from build123d import *

# Parameters (mm, degrees)
SCHIZZO1_W                   = 170
SCHIZZO1_H                   = 55
ESTRUSIONE_ESTRUSIONE2_DEPTH = 5
SCHIZZO2_W                   = 15
SCHIZZO2_H                   = 5
TAGLIO_ESTRUSIONE1_DEPTH     = 6
TAGLIO_ESTRUSIONE3_DEPTH     = 6


with BuildPart() as part:
    # Schizzo1 → Estrusione-Estrusione2 (new body)
    with BuildSketch(Plane(origin=(0, 0, 0), x_dir=(1, 0, 0), z_dir=(0, 1, 0))):
        with Locations((30.43505086, -0.781075862)):
            Rectangle(SCHIZZO1_W, SCHIZZO1_H)
    extrude(amount=-ESTRUSIONE_ESTRUSIONE2_DEPTH)

    # Schizzo2 → Taglio-Estrusione1 (cut, through all)
    with BuildSketch(Plane(origin=(0, 0, 0), x_dir=(1, 0, 0), z_dir=(0, 1, 0))):
        with Locations((-47.06494914, -25.781075862)):
            Rectangle(SCHIZZO2_W, SCHIZZO2_H)
        with Locations((-47.06494914, 24.218924138)):
            Rectangle(SCHIZZO2_W, SCHIZZO2_H)
        with Locations((107.93505086, -25.781075862)):
            Rectangle(SCHIZZO2_W, SCHIZZO2_H)
        with Locations((107.93505086, 24.218924138)):
            Rectangle(SCHIZZO2_W, SCHIZZO2_H)
        with Locations((30.43505086, -25.781075862)):
            Rectangle(SCHIZZO2_W, SCHIZZO2_H)
        with Locations((30.43505086, 24.218924138)):
            Rectangle(SCHIZZO2_W, SCHIZZO2_H)
    extrude(amount=-TAGLIO_ESTRUSIONE1_DEPTH, mode=Mode.SUBTRACT)

    # Schizzo3 → Taglio-Estrusione3 (cut, through all)
    with BuildSketch(Plane(origin=(0, 0, 0), x_dir=(1, 0, 0), z_dir=(0, 1, 0))):
        Polygon((-48.56494914, -23.281075862), (-45.56494914, -23.281075862), (-45.56494914, -16.281075862), (-42.22494914, -16.281075862), (-42.22494914, -13.281075862), (-45.56494914, -13.281075862), (-45.56494914, -5.281075862), (-48.56494914, -5.281075862), (-48.56494914, -13.281075862), (-51.90494914, -13.281075862), (-51.90494914, -16.281075862), (-48.56494914, -16.281075862), align=None)
        Polygon((28.93505086, -23.281075862), (31.93505086, -23.281075862), (31.93505086, -16.281075862), (35.27505086, -16.281075862), (35.27505086, -13.281075862), (31.93505086, -13.281075862), (31.93505086, -5.281075862), (28.93505086, -5.281075862), (28.93505086, -13.281075862), (25.59505086, -13.281075862), (25.59505086, -16.281075862), (28.93505086, -16.281075862), align=None)
        Polygon((106.43505086, -23.281075862), (109.43505086, -23.281075862), (109.43505086, -16.281075862), (112.77505086, -16.281075862), (112.77505086, -13.281075862), (109.43505086, -13.281075862), (109.43505086, -5.281075862), (106.43505086, -5.281075862), (106.43505086, -13.281075862), (103.09505086, -13.281075862), (103.09505086, -16.281075862), (106.43505086, -16.281075862), align=None)
        Polygon((106.43505086, 3.718924138), (109.43505086, 3.718924138), (109.43505086, 11.718924138), (112.77505086, 11.718924138), (112.77505086, 14.718924138), (109.43505086, 14.718924138), (109.43505086, 21.718924138), (106.43505086, 21.718924138), (106.43505086, 14.718924138), (103.09505086, 14.718924138), (103.09505086, 11.718924138), (106.43505086, 11.718924138), align=None)
        Polygon((28.93505086, 3.718924138), (31.93505086, 3.718924138), (31.93505086, 11.718924138), (35.27505086, 11.718924138), (35.27505086, 14.718924138), (31.93505086, 14.718924138), (31.93505086, 21.718924138), (28.93505086, 21.718924138), (28.93505086, 14.718924138), (25.59505086, 14.718924138), (25.59505086, 11.718924138), (28.93505086, 11.718924138), align=None)
        Polygon((-48.56494914, 3.718924138), (-45.56494914, 3.718924138), (-45.56494914, 11.718924138), (-42.22494914, 11.718924138), (-42.22494914, 14.718924138), (-45.56494914, 14.718924138), (-45.56494914, 21.718924138), (-48.56494914, 21.718924138), (-48.56494914, 14.718924138), (-51.90494914, 14.718924138), (-51.90494914, 11.718924138), (-48.56494914, 11.718924138), align=None)
    extrude(amount=-TAGLIO_ESTRUSIONE3_DEPTH, mode=Mode.SUBTRACT)


solid = part.part
Could you check a few things on this model? Use its own coordinates, in mm. A direction names the side the tool comes from. Give positions to 0.01 mm unless a question says otherwise; leave off trailing zeros. Write each loop counter-clockwise with the first axis right and the second up, starting at its lowest first coordinate (ties: lowest second). Pieces come first, ordered by that corner, then holes. Notation, with made-up numbers: (2.25, -4.5) -> (9.25, -4.5) arc R24 ccw to (9.25, 17.5) -> close; hole circle Ø2 at (1, -33). An arc over 180 degrees is marked (long way). Write each question's results on one line, items separated by ' | '. Start each with the question number.
Q1. I need wall thicknesses on probe 1 along X at (y, z) = (-2.15, -21); probe 2 along X at (y, z) = (-4.35, 16); probe 3 along Z at (x, y) = (27.5, -4.15). Which ranges of each line are inside material? Lowest first, please.
Q2. Which directions (+Z, -Z, +X, -X, +Y, -Y) give clear straight access to the entire face, cutting with the end or side of a thin tool? Please do faces 1 (the face through (-43, -2, -21.719)), 2 (the face through (111, -2, 16.281)), 3 (the face through (-39.565, -2, 26)).
Q3. Suppose I cut it at A-A, the plane z = 9.5. List the corners of the cut face in (x, y) for me, and give its area (3 significant figures).
Q4. I'm going to push a flat-ended pin straight in: pin 1 Ø1.7 at (x, y) = (-51, -3.5) entering from -Z. Where does the tip first touch, or does it pass through?
Outcome:
1) probe 1: -54.56 to -48.56, -45.56 to 28.94, 31.94 to 106.44, 109.44 to 115.44 | probe 2: -54.56 to -51.9, -42.22 to 25.6, 35.28 to 103.1, 112.78 to 115.44 | probe 3: -21.72 to -14.72, -11.72 to 13.28, 16.28 to 23.28
2) face 1: -Z, -X, +Y, -Y | face 2: +Y, -Y | face 3: +Z, -X, +Y, -Y
3) outline: (-54.56, -5) -> (-48.56, -5) -> (-48.56, 0) -> (-54.56, 0) -> close; (-45.56, -5) -> (28.94, -5) -> (28.94, 0) -> (-45.56, 0) -> close; (31.94, -5) -> (106.44, -5) -> (106.44, 0) -> (31.94, 0) -> close; (109.44, -5) -> (115.44, -5) -> (115.44, 0) -> (109.44, 0) -> close | area: 805 mm2
4) pin 1: z = -21.72
